from build123d import *

# Parameters (mm, degrees)
SKETCH_1_W          = 28
SKETCH_1_H          = 18
EXTRUDE_1_DEPTH     = 40
SKETCH_2_R          = 2
CUT_EXTRUDE_1_DEPTH = 15
SKETCH_4_R          = 7.5
CUT_EXTRUDE_2_DEPTH = 1.2
SKETCH_5_R          = 6.5
CUT_EXTRUDE_3_DEPTH = 3.2
CUT_EXTRUDE_4_REACH = 51.809
SKETCH_6_R          = 2.5
CUT_EXTRUDE_START   = -1.2
SKETCH_7_R          = 7.5
CUT_EXTRUDE_5_DEPTH = 1.2
CUT_EXTRUDE_START_2 = -3.2
SKETCH_8_R          = 6.5
CUT_EXTRUDE_6_DEPTH = 3.2
CUT_EXTRUDE_7_DEPTH = 53.038447325
EXTRUDE_START       = 1.2
SKETCH_10_R         = 7.5
SKETCH_10_R_2       = 6.5
EXTRUDE_2_DEPTH     = 1.2
SKETCH_11_R         = 7.5
SKETCH_11_R_2       = 6.5
EXTRUDE_3_DEPTH     = 1.2
CUT_EXTRUDE_START_3 = -19.2
SKETCH_12_R         = 6.5
CUT_EXTRUDE_8_DEPTH = 19.2


with BuildPart() as part:
    # 草图1 → 凸台-拉伸1 (new body)
    with BuildSketch(Plane(origin=(0, 0, 0), x_dir=(1, 0, 0), z_dir=(0, 1, 0))):
        with Locations((14, 9)):
            Rectangle(SKETCH_1_W, SKETCH_1_H)
    extrude(amount=EXTRUDE_1_DEPTH)

    # 草图2 → 切除-拉伸1 (cut)
    with BuildSketch(Plane.XZ):
        with Locations(Location((6, -5.5, 0), (0, 0, 270))):
            Circle(SKETCH_2_R)
        with Locations(Location((6, -12.5, 0), (0, 0, 270))):
            Circle(SKETCH_2_R)
        with Locations(Location((22, -12.5, 0), (0, 0, 90))):
            Circle(SKETCH_2_R)
        with Locations(Location((22, -5.5, 0), (0, 0, 90))):
            Circle(SKETCH_2_R)
    extrude(amount=-CUT_EXTRUDE_1_DEPTH, mode=Mode.SUBTRACT)

    # 草图4 → 切除-拉伸2 (cut)
    with BuildSketch(Plane(origin=(28, 0, 0), x_dir=(0, 0, -1), z_dir=(1, 0, 0))):
        with Locations((9, 28.5)):
            Circle(SKETCH_4_R)
    extrude(amount=-CUT_EXTRUDE_2_DEPTH, mode=Mode.SUBTRACT)

    # 草图5 → 切除-拉伸3 (cut)
    with BuildSketch(Plane(origin=(26.8, 0, 0), x_dir=(0, 0, -1), z_dir=(1, 0, 0))):
        with Locations((9, 28.5)):
            Circle(SKETCH_5_R)
    extrude(amount=-CUT_EXTRUDE_3_DEPTH, mode=Mode.SUBTRACT)

    # 草图6 → 切除-拉伸4 (cut, up to next)
    with BuildSketch(Plane(origin=(23.6, 0, 0), x_dir=(0, 0, -1), z_dir=(1, 0, 0)), mode=Mode.PRIVATE) as cut_extrude_4_sk1:
        with Locations((9, 28.5)):
            Circle(SKETCH_6_R)
    cut_extrude_4_tool1 = extrude(cut_extrude_4_sk1.sketch, amount=-CUT_EXTRUDE_4_REACH, mode=Mode.PRIVATE) & part.part
    add(cut_extrude_4_tool1.solids().sort_by_distance((23.6, 28.5, -9))[0], mode=Mode.SUBTRACT)

    # 草图7 → 切除-拉伸5 (cut)
    with BuildSketch(Plane.ZY.offset(CUT_EXTRUDE_START)):
        with Locations(Location((-9, 28.5, 0), (0, 0, 180))):
            Circle(SKETCH_7_R)
    extrude(amount=CUT_EXTRUDE_5_DEPTH, mode=Mode.SUBTRACT)

    # 草图8 → 切除-拉伸6 (cut)
    with BuildSketch(Plane.ZY.offset(-1.2).offset(CUT_EXTRUDE_START_2)):
        with Locations(Location((-9, 28.5, 0), (0, 0, 180))):
            Circle(SKETCH_8_R)
    extrude(amount=CUT_EXTRUDE_6_DEPTH, mode=Mode.SUBTRACT)

    # 草图9 → 切除-拉伸7 (cut, through all)
    with BuildSketch(Plane.XY):
        Polygon((14, 40), (11.5, 40), (11.5, 20), (16.5, 20), (16.5, 40), align=None)
    extrude(amount=-CUT_EXTRUDE_7_DEPTH, mode=Mode.SUBTRACT)

    # 草图10 → 凸台-拉伸2 (add)
    with BuildSketch(Plane(origin=(26.8, 0, 0), x_dir=(0, 0, -1), z_dir=(1, 0, 0)).offset(EXTRUDE_START)):
        with Locations(Location((9, 28.5, 0), (0, 0, 180))):
            Circle(SKETCH_10_R)
        with Locations((9, 28.5)):
            Circle(SKETCH_10_R_2, mode=Mode.SUBTRACT)
    extrude(amount=-EXTRUDE_2_DEPTH)

    # 草图11 → 凸台-拉伸3 (add)
    with BuildSketch(Plane.ZY.offset(-1.2)):
        with Locations((-9, 28.5)):
            Circle(SKETCH_11_R)
        with Locations(Location((-9, 28.5, 0), (0, 0, 180))):
            Circle(SKETCH_11_R_2, mode=Mode.SUBTRACT)
    extrude(amount=EXTRUDE_3_DEPTH)

    # 草图12 → 切除-拉伸8 (cut)
    with BuildSketch(Plane.ZY.offset(-4.4).offset(CUT_EXTRUDE_START_3)):
        with Locations(Location((-9, 28.5, 0), (0, 0, 180))):
            Circle(SKETCH_12_R)
    extrude(amount=CUT_EXTRUDE_8_DEPTH, mode=Mode.SUBTRACT)


solid = part.part
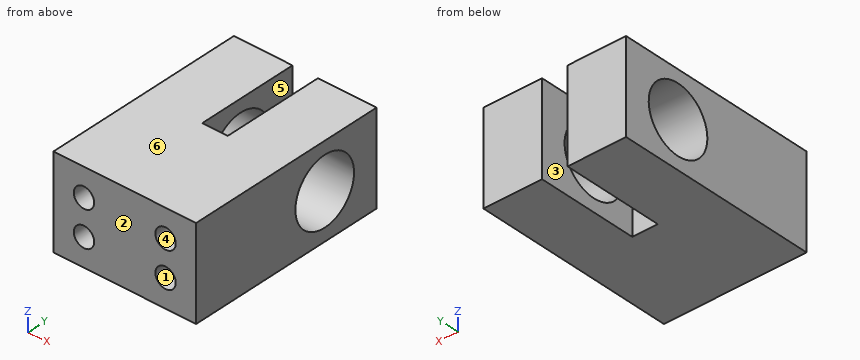
Could you check a few things on this model? Use its own coordinates, in mm. Face numbers are marked on the shaded views. A direction names the side the tool comes from. Give positions to 0.01 mm unless a question says otherwise; leave off trailing zeros. Order: outer loops, then holes, each group sorted by start corner. A loop starts at its lowest first (then second) coordinate and runs counter-clockwise, first axis right, second up. Notation, with made-up numbers: M 52.5,84.25 L 61.5,84.25 A19 cw 61.5,119.25 Z; hole C 35,84.25 d7. An arc over 180 degrees is marked long. One line per question, with ' | ' between items.
1. I want a section at A-A (y = 28.5). List the corners of the cut face in (x, z) for me, and give its area (3 significant figures).
Results:
outline: M 0,-18 L 11.5,-18 L 11.5,-15.5 L 0,-15.5 Z; M 0,-2.5 L 11.5,-2.5 L 11.5,0 L 0,0 Z; M 16.5,-18 L 28,-18 L 28,-15.5 L 16.5,-15.5 Z; M 16.5,-2.5 L 28,-2.5 L 28,0 L 16.5,0 Z | area: 115 mm²
2. If I drill on line 1 (X direction, y = 8, z = -5.5); line 2 (Z direction, x = 22, y = 3); line 3 (Z direction, x = 23.5, y = 11), over which ranges is the centre line in solid material (lowest first)?
Results:
line 1: 0 to 4, 8 to 20, 24 to 28 | line 2: -18 to -14.5, -10.5 to -7.5, -3.5 to 0 | line 3: -18 to -13.82, -11.18 to -6.82, -4.18 to 0
3. I want a section at C-C (x = 6). List the corners of the cut face in (y, z) for me, and give its area (3 significant figures).
Results:
outline: M 0,-18 L 40,-18 L 40,0 L 0,0 L 0,-3.5 L 15,-3.5 L 15,-7.5 L 0,-7.5 L 0,-10.5 L 15,-10.5 L 15,-14.5 L 0,-14.5 Z; hole C 28.5,-9 d13 | area: 467 mm²
4. I'm going to push flat-ended pins straight in: pin 1 (4 mm diameter, centred on x = 14, z = -12.5, fed in from +Y); pin 2 (3 mm diameter, centred on x = 6, z = -12.5, fed in from -Y). Where does each tip first touch, or does it pass through?
Results:
pin 1: y = 20 | pin 2: y = 15
5. I want a section at B-B (z = -9). List the corners of the cut face in (x, y) for me.
Results:
outline: M 0,0 L 28,0 L 28,22 L 16.5,22 L 16.5,20 L 11.5,20 L 11.5,22 L 0,22 Z; M 0,35 L 11.5,35 L 11.5,40 L 0,40 Z; M 16.5,35 L 28,35 L 28,40 L 16.5,40 Z
6. We'd pull the mould along Z, two halves only. Please class the marked faces 4, 5 and 6: +Z half, -Z half, draft (parallel to the pull), parting line (faces both ways), or undercut.
Results:
face 4: undercut | face 5: draft | face 6: +Z half
7. I want a section at D-D (y = 6). List the corners of the cut face in (x, z) for me.
Results:
outline: M 0,-18 L 28,-18 L 28,0 L 0,0 Z; hole C 6,-12.5 d4; hole C 6,-5.5 d4; hole C 22,-12.5 d4; hole C 22,-5.5 d4
8. For the marked faces 1, 2 and 3, which set-ups out of +Z, -Z, +X, -X, +Y, -Y let a thin tool reach every point of the face, with its end or its side?
Results:
face 1: -Y | face 2: +Z, -Z, +X, -X, -Y | face 3: +Z, -Z, +Y
